Autodesk Inventor part; units mm, degrees
ref_plane "Work Plane3" through (38.0048, 15, 0) normal (1, 0, 0) x (0, 1, 0)
ref_plane "Work Plane5" through (0, 15, 0) normal (-1, 0, 0) x (0, -1, 0)
ref_plane "Work Plane6" through (0, 15, 38.0048) normal (0, 0, 1) x (1, 0, 0)
sketch "Sketch1" plane through (0, 0, 0) normal (0, 1, 0) x (-1, 0, 0)
  circle A0 centre (0, 0) radius 44.45
  circle A1 centre (0, 0) radius 6.75
  dimension "d0" = 88.9
  dimension "d3" = 13.5
extrude "Extrusion2" add sketch "Sketch1" along normal blind 2 contours A0 | A1
sketch "Sketch2" plane through (0, 2, 0) normal (0, 1, 0) x (1, 0, 0)
  circle A0 centre (0, 0) radius 10
  circle A1 centre (0, 0) radius 44.45
  dimension "d6" = 20
  dimension "d37" = 88.9
extrude "Extrusion3" add sketch "Sketch2" along normal blind 7 contours A0 | A1
sketch "Sketch3" plane through (0, 9, 0) normal (0, 1, 0) x (1, 0, 0)
  circle A0 centre (0, 0) radius 44.45
  dimension "d9" = 88.9
extrude "Extrusion4" add sketch "Sketch3" along normal blind 6
sketch "Sketch4" plane through (0, 15, 0) normal (0, 1, 0) x (1, 0, 0)
  circle A0 centre (0, 0) radius 38.0048
  circle A1 centre (0, 0) radius 31.75
  point P0 (-38.0048, 0)
  point P1 (0, 38.0048)
  point P2 (38.0048, 0)
  point P3 (0, -38.0048)
  dimension "d12" = 76.0095
  dimension "d13" = 63.5
extrude "Extrusion5" add sketch "Sketch4" along normal blind 31.75
ref_plane "Work Plane3" through (38.0048, 15, 0) normal (1, 0, 0) x (0, 1, 0)
ref_plane "Work Plane4" through (-38.0048, 15, 0) normal (-1, 0, 0) x (0, -1, 0)
sketch "Sketch8" plane through (38.0048, 15, 0) normal (1, 0, 0) x (0, 1, 0)
  line L0 (31.75, -38.0048) -> (31.75, 38.0048)
  line L1 (31.75, 6.35) -> (14.224, 6.35)
  line L2 (14.224, 6.35) -> (14.224, -6.35)
  line L3 (14.224, -6.35) -> (31.75, -6.35)
  line L4 (31.75, -6.35) -> (31.75, 6.35)
  line L5 (31.75, 0) -> (0, 0)
  line L6 (0, -44.45) -> (0, 44.45)
  line L7 (21.844, 5.08) -> (17.4498, 5.08)
  line L8 (17.4498, 5.08) -> (17.4498, -5.08)
  line L9 (17.4498, -5.08) -> (21.844, -5.08)
  line L10 (21.844, -5.08) -> (21.844, 5.08)
  line L11 (25.146, 6.35) -> (25.146, -6.35)
  point P0 (-15, 0)
  dimension "d38" = 17.526
  dimension "d39" = 12.7
  dimension "d41" = 6.35
  dimension "d42" = 9.906
  dimension "d43" = 10.16
  dimension "d44" = 5.08
  dimension "d46" = 4.3942
  dimension "d70" = 6.604
extrude "Extrusion9" [suppressed]
ref_plane "Work Plane5" through (0, 15, 0) normal (-1, 0, 0) x (0, -1, 0)
mirror "Mirror1" [suppressed]
fillet "Fillet3" [suppressed]
fillet "Fillet4" [suppressed]
fillet "Fillet5" [suppressed]
fillet "Fillet6" [suppressed]
sketch "Sketch9" plane through (0, 15, 0) normal (0, 1, 0) x (1, 0, 0)
  line L0 (-9, 0.8983) -> (-5, 0.8983)
  line L1 (-9.0449, -0.0017) -> (-5, -0.0017)
  line L2 (-5, -0.0017) -> (-5, 0.8983)
  circle A0 centre (0, -0.0017) radius 9.0449
  circle A1 centre (0, -0.0017) radius 21.8449
  line L3 (-21.8449, 0) -> (-25.8449, 0)
  circle A2 centre (0, -0.0017) radius 25.8449
  point P0 (0, 0)
  dimension "d62" = 43.6898
  dimension "d57" = 4
  dimension "d58" = 5
  dimension "d60" = 0.9
  dimension "x" = 18.0898
  dimension "d63" = 4
extrude "Extrusion10" cut sketch "Sketch9" against normal blind 12 contours L0 L2 L1 A0 | A1 | A2 picked at (-6.3416, 0.4985)
sketch "Sketch10" plane through (0, 15, 0) normal (0, 1, 0) x (1, 0, 0)
  circle A0 centre (0, 0) radius 2.3178
  dimension "d67" = 4.6355
extrude "Extrusion11" add sketch "Sketch10" along normal blind 4.064
ref_plane "Work Plane6" through (0, 15, 38.0048) normal (0, 0, 1) x (1, 0, 0)
sketch "Sketch11" plane through (0, 15, 38.0048) normal (0, 0, 1) x (1, 0, 0)
  line L0 (-31.75, 31.75) -> (31.75, 31.75)
  line L1 (0, 31.75) -> (0, 22.225)
  line L2 (-4.7625, 22.225) -> (4.7625, 22.225)
  line L3 (4.7625, 22.225) -> (4.7625, 31.75)
  line L4 (4.7625, 31.75) -> (-4.7625, 31.75)
  line L5 (-4.7625, 31.75) -> (-4.7625, 22.225)
  point P0 (0, -15)
  point P1 (-4.7625, 31.75)
  dimension "d71" = 9.525
  dimension "d72" = 4.7625
  dimension "d73" = 4.7625
extrude "Extrusion12" cut sketch "Sketch11" against normal blind 100.0872
sketch "Sketch12" plane through (0, 0, 0) normal (0, -1, 0) x (1, 0, 0)
  circle A0 centre (0, 0) radius 1.5
  dimension "d76" = 3
extrude "Extrusion13" cut sketch "Sketch12" against normal blind 8
thread "Thread2"
properties part number "LidBottom"
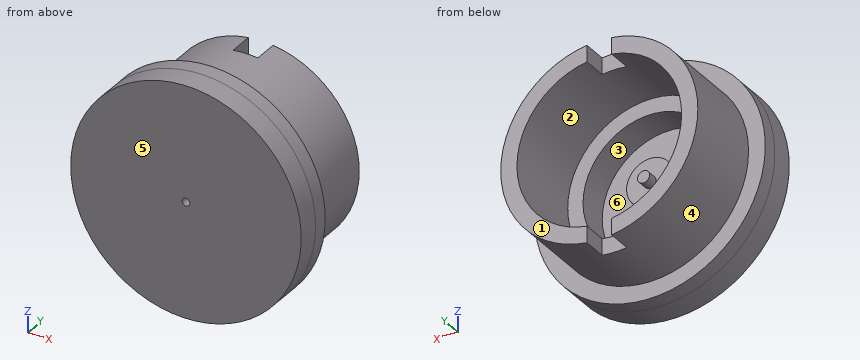
Check sheet for the modelled part. Datum: model origin and axes. Units: mm. Face numbers are marked on the shaded views. A direction names the side the tool comes from. Round coordinates to 2 decimals unless told otherwise and drop trailing zeros. Order: outer loops, then holes, each group sorted by start corner. A loop starts at its lowest first (then second) coordinate and runs counter-clockwise, first axis right, second up. Notation, with made-up numbers: (-32, 29) -> (14, 29) arc R22 cw to (14, 39) -> close; hole circle Ø4 at (-39, 29). An arc over 180 degrees is marked (long way). One line per item, written item: value. Start each with the question number.
Q1. Gauge pin test, flat ends, axial feed: pin 1 Ø3 at (y, z) = (31, -1.5) entering from -X; pin 2 Ø10 at (y, z) = (12.5, 16) entering from +X; pin 3 Ø2.5 at (x, z) = (0, 0) entering from +Y; pin 4 Ø2.5 at (x, z) = (-0.5, 0.5) entering from -Y. Record the tip position at first contact, or that the pin passes through.
Q2. Mould release check, pull along X, two halves, no side actions. Record for the marked faces 3, 4, 5 and 6: pulls with the +X half, pulls with the -X half, needs draft (parallel to the pull), parting line crosses it, or undercut.
Q3. Cross-section at A-A (y = 13). Record the boundary of the cut face in (x, z).
Q4. Cross-section at D-D (z = -21). Record the boundary of the cut face in (x, y).
Q5. Set-up check for the marked faces 1 and 2: record each of +Z, -Z, +X, -X, +Y, -Y from which the full face is reachable in a straight line by a thin tool's end or side.
Q6. Thickness scan on line 1 (Z direction, x = 0, y = 6.75); line 2 (Z direction, x = 0, y = 9); line 3 (X direction, y = 39.5, z = 0). Record the ranges inside material, lowest first.
Q7. Cross-section at C-C (y = 30). Record the boundary of the cut face in (x, z).
Completed:
1. pin 1: stops at x = -38
1. pin 2: stops at x = 43.07
1. pin 3: stops at y = 19.06
1. pin 4: stops at y = 0
2. face 3: undercut
2. face 4: parting line crosses it
2. face 5: needs draft
2. face 6: undercut
3. outline: circle Ø88.9 at (0, 0); (-9.04, 0) -> (-5, 0) -> (-5, -0.9) -> (-9, -0.9) arc R9.04 ccw (long way) to start; hole circle Ø51.69 at (0, 0)
4. outline: (-39.18, 0) -> (39.18, 0) -> (39.18, 15) -> (31.68, 15) -> (31.68, 46.75) -> (23.81, 46.75) -> (23.81, 15) -> (15.06, 15) -> (15.06, 3) -> (-15.06, 3) -> (-15.06, 15) -> (-23.81, 15) -> (-23.81, 46.75) -> (-31.68, 46.75) -> (-31.68, 15) -> (-39.18, 15) -> close
5. face 1: +Z, -Z, +X, -X, +Y
5. face 2: +Y
6. line 1: z = -44.45 to -25.84, -9.04 to -1.5, 1.5 to 9.05, 25.85 to 44.45
6. line 2: z = -44.45 to -25.84, -9.04 to 9.05, 25.85 to 44.45
6. line 3: x = -38 to -31.75, 31.75 to 38
7. outline: circle Ø76.01 at (0, 0); hole circle Ø63.5 at (0, 0)
